```python
from build123d import *

# Parameters (mm, degrees)
EXTRUDE_1_DEPTH          = 22
CUT_EXTRUDE_START        = -4
CUT_EXTRUDE_1_DEPTH      = 4
SKETCH_3_W               = 2
SKETCH_3_H               = 1.5
CUT_EXTRUDE_2_DEPTH      = 5
FILLET_1_R               = 7
CUT_EXTRUDE_3_DEPTH      = 55.478956816
CUT_EXTRUDE_3_DEPTH_BACK = 55.478956816
SKETCH_11_W              = 74.866363777
SKETCH_11_H              = 10.751937883
CUT_EXTRUDE_4_DEPTH      = 43.459689965
CUT_EXTRUDE_4_DEPTH_BACK = 43.459689965
SKETCH_12_R              = 1.6


with BuildPart() as part:
    # 草图1 → 凸台-拉伸1 (new body)
    with BuildSketch(Plane.XY.offset(11)):
        with BuildLine():
            Line((22.242183112, 32.436253827), (14.268783679, 32.436253827))
            Line((14.268783679, 32.436253827), (14.268783679, 3.77031158))
            Line((14.268783679, 3.77031158), (-9.293805711, -12.555760396))
            ThreePointArc((-9.293805711, -12.555760396), (-11.060906945, -22.296261062), (-1.320406278, -24.063362296))
            Line((-1.320406278, -24.063362296), (22.242183112, -7.73729032))
            Line((22.242183112, -7.73729032), (22.242183112, 32.436253827))
        make_face()
    extrude(amount=-EXTRUDE_1_DEPTH)

    # 草图2 → 切除-拉伸1 (cut)
    with BuildSketch(Plane(origin=(0, 0, -11), x_dir=(-1, 0, 0), z_dir=(0, 0, -1)).offset(CUT_EXTRUDE_START)):
        with BuildLine():
            Line((6.652022195, -14.542440374), (-11.373854522, -8.10694393))
            Line((-11.373854522, -8.10694393), (-11.878198097, -9.519614294))
            Line((-11.878198097, -9.519614294), (3.206970754, -14.905235866))
            ThreePointArc((3.206970754, -14.905235866), (1.308519825, -18.203219238), (3.028991871, -21.597447603))
            Line((3.028991871, -21.597447603), (1.320406278, -24.063362296))
            ThreePointArc((1.320406278, -24.063362296), (8.554651374, -24.510645848), (12.307105995, -18.309561346))
            Line((12.307105995, -18.309561346), (9.307105995, -18.309561346))
            ThreePointArc((9.307105995, -18.309561346), (8.576636909, -16.005181256), (6.652022195, -14.542440374))
        make_face()
    extrude(amount=CUT_EXTRUDE_1_DEPTH, mode=Mode.SUBTRACT)

    # 草图3 → 切除-拉伸2 (cut)
    with BuildSketch(Plane(origin=(7.520945342, 2.685085323, 0), x_dir=(0, 0, 1), z_dir=(-0.9417802429021499, -0.3362290500227003, 0))):
        with Locations((-8, -12.209179925)):
            Rectangle(SKETCH_3_W, SKETCH_3_H)
    extrude(amount=-CUT_EXTRUDE_2_DEPTH, mode=Mode.SUBTRACT)

    # 圆角1
    fillet_1_edges = [part.edges().sort_by_distance(p)[0] for p in [
        (22.242183112, -7.73729032, 0),
        (14.268783679, 3.77031158, 0),
    ]]
    fillet(fillet_1_edges, radius=FILLET_1_R)

    # 草图11 → 切除-拉伸3 (cut, two sides: drawn at the far end of the back side and taken through both)
    with BuildSketch(Plane(origin=(10.836641759, -15.639973933, 0), x_dir=(0.8219715642635482, 0.5695285309289919, 0), z_dir=(0.5695285309289919, -0.8219715642635482, 0)).offset(-CUT_EXTRUDE_3_DEPTH_BACK)):
        with Locations((13.262652651, 10.375968942)):
            Rectangle(SKETCH_11_W, SKETCH_11_H)
    extrude(amount=CUT_EXTRUDE_3_DEPTH + CUT_EXTRUDE_3_DEPTH_BACK, mode=Mode.SUBTRACT)

    # 草图12 → 切除-拉伸4 (cut, two sides: drawn at the far end of the back side and taken through both)
    with BuildSketch(Plane.XY.offset(5).offset(-CUT_EXTRUDE_4_DEPTH_BACK)):
        with Locations(Location((-5.307105995, -18.309561346, 0), (0, 0, 180))):
            Circle(SKETCH_12_R)
        with Locations((16.17499904, -3.425017581)):
            Circle(SKETCH_12_R)
    extrude(amount=CUT_EXTRUDE_4_DEPTH + CUT_EXTRUDE_4_DEPTH_BACK, mode=Mode.SUBTRACT)


solid = part.part
```
Build history of the part. All positions in model axes, mm. A direction names the side the tool comes from. Round coordinates to 2 decimals unless told otherwise and drop trailing zeros. Write each loop counter-clockwise with the first axis right and the second up, starting at its lowest first coordinate (ties: lowest second). Pieces come first, ordered by that corner, then holes.
1) Pin check, flat tips, straight feed: pin 1 (6 mm diameter, centred on y = -3, z = -3, fed in from -X); pin 2 (6 mm diameter, centred on y = -9.5, z = -7.5, fed in from -X); pin 3 (2 mm diameter, centred on x = 0.5, z = -7, fed in from +Y). Stop position of each tip, or through.
2) Mould opens along X. For faces 5 (the flat face through (8.81, -17.044, -2.888)), 6 (the cylindrical face through (-5.099, -19.896, -1.084)), 7 (the cylindrical face through (13.49, 4.23, -3.11)) say: +X half, -X half, draft (parallel to the pull), parting line (faces both ways), or undercut.
3) Band-saw the part on A-A, the plane z = 0.5. List the corners of the cut face in (x, y) (3 decimals), and give its area (3 significant figures).
4) Drill centre lines: probe 1 along X at (y, z) = (7.5, 3.25); probe 2 along Z at (x, y) = (-7, -23); probe 3 along Y at (x, z) = (15, 1.75). Where is each one in solid material? Low to high.
5) Band-saw the part on C-C, the plane y = 27. List the corners of the cut face in (x, z), and give its area (3 significant figures).
6) Band-saw the part on B-B, the plane x = -5. List the corners of the cut face in (y, z), and give its area (3 significant figures).
7) 3-axis set-ups, long thin cutter, end or side, ignore diameter. For faces 1 (the flat face through (14, -8, -9)), 2 (the flat face through (-11, -18.31, -9)), 3 (the flat face through (14.269, 20, -3)), 4 (the cylindrical face through (-8.596, -16.033, -8.972)): which of +Z, -Z, +X, -X, +Y, -Y reach the whole face in a straight line?
8) Band-saw the part on D-D, the plane z = -8.25. List the corners of the cut face in (x, y) (3 decimals).
Ans:
1. pin 1: stops at x = 0.17
1. pin 2: stops at x = -9.21
1. pin 3: stops at y = -5.08
2. face 5: +X half
2. face 6: undercut
2. face 7: -X half
3. outline: (-9.294, -12.556) arc R7 ccw to (-1.32, -24.063) - (19.229, -9.825) arc R7 ccw to (22.242, -4.071) - (22.242, 32.436) - (14.269, 32.436) - (14.269, 7.436) arc R7 cw to (11.255, 1.682) - close; hole circle Ø3.2 at (-5.307, -18.31); hole circle Ø3.2 at (16.175, -3.425)
3. area: 737 mm2
4. probe 1: x = 14.27 to 22.24
4. probe 2: z = -7 to 5
4. probe 3: y = -12.76 to -4.51, -2.34 to 32.44
5. outline: (14.27, -11) - (22.24, -11) - (22.24, 5) - (14.27, 5) - close
5. area: 128 mm2
6. outline: (-25.3, -7) - (-19.88, -7) - (-19.88, 5) - (-25.3, 5) - close; (-16.74, -7) - (-13.95, -7) - (-13.95, -11) - (-9.58, -11) - (-9.58, 5) - (-16.74, 5) - close
6. area: 168 mm2
7. face 1: none
7. face 2: -Z, -X, -Y
7. face 3: +Z, -Z, -X, +Y
7. face 4: -Z, -Y
8. outline: (-12.307, -18.31) - (-9.307, -18.31) arc R4 cw to (-6.652, -14.542) - (16.083, -6.426) - (16.587, -7.838) - (-3.207, -14.905) arc R4 cw to (-3.029, -21.597) - (-1.32, -24.063) - (19.229, -9.825) arc R7 ccw to (22.242, -4.071) - (22.242, 32.436) - (14.269, 32.436) - (14.269, 7.436) arc R7 cw to (11.255, 1.682) - (-9.294, -12.556) arc R7 ccw to start; hole circle Ø3.2 at (16.175, -3.425)
